Geometry check sheet. Reference: the model listing, model coordinates, mm. A direction names the side the tool comes from. Coordinates: 2 decimals unless noted, no trailing zeros. Write each loop counter-clockwise with the first axis right and the second up, starting at its lowest first coordinate (ties: lowest second). Pieces come first, ordered by that corner, then holes.
from build123d import *

# Parameters (mm, degrees)
SKETCH_1_W                      = 6
SKETCH_1_H                      = 20
EXTRUDE_1_DEPTH                 = 165
HOLE_WIZARD_G1_16_1_D           = 6.6
HOLE_WIZARD_G1_16_1_DEPTH       = 50
HOLE_WIZARD_G1_16_1_CSINK_D     = 7.773
HOLE_WIZARD_G1_16_1_CSINK_ANGLE = 90
HOLE_WIZARD_G1_16_1_TIP         = 1.982840043
SKETCH_5_W                      = 15
SKETCH_5_H                      = 20
EXTRUDE_2_DEPTH                 = 10
EXTRUDE_2_DEPTH_BACK            = 15
SKETCH_6_W                      = 5.5
SKETCH_6_H                      = 15
SKETCH_6_W_2                    = 4.5
CUT_EXTRUDE_1_DEPTH             = 32
SKETCH_7_W                      = 15
SKETCH_7_H                      = 18
CUT_EXTRUDE_2_DEPTH             = 14
SKETCH_8_R                      = 2
CUT_EXTRUDE_3_DEPTH             = 39
CUT_EXTRUDE_4_DEPTH             = 70


with BuildPart() as part:
    # 草图1 → 凸台-拉伸1 (new body)
    with BuildSketch(Plane.XY):
        Rectangle(SKETCH_1_W, SKETCH_1_H)
    extrude(amount=EXTRUDE_1_DEPTH)

    # G1/16 螺纹孔1
    with Locations(Plane(origin=(3, 0, 0), x_dir=(0, 0, -1), z_dir=(1, 0, 0))):
        with Locations((-5, 0)):
            CounterSinkHole(HOLE_WIZARD_G1_16_1_D / 2, HOLE_WIZARD_G1_16_1_CSINK_D / 2, depth=HOLE_WIZARD_G1_16_1_DEPTH, counter_sink_angle=HOLE_WIZARD_G1_16_1_CSINK_ANGLE)
            with Locations((0, 0, -(HOLE_WIZARD_G1_16_1_DEPTH + HOLE_WIZARD_G1_16_1_TIP / 2))):  # 118° drill point
                Cone(0, HOLE_WIZARD_G1_16_1_D / 2, HOLE_WIZARD_G1_16_1_TIP, mode=Mode.SUBTRACT)

    # 草图5 → 凸台-拉伸2 (add, two sides)
    with BuildSketch(Plane(origin=(3, 0, 0), x_dir=(0, 0, -1), z_dir=(1, 0, 0))) as extrude_2_sk:
        with Locations((-160.5, 0)):
            Rectangle(SKETCH_5_W, SKETCH_5_H)
    extrude(amount=EXTRUDE_2_DEPTH)
    extrude(extrude_2_sk.sketch, amount=-EXTRUDE_2_DEPTH_BACK)

    # 草图6 → 切除-拉伸1 (cut)
    with BuildSketch(Plane.XZ.offset(10)):
        with Locations((10.25, 160.5)):
            Rectangle(SKETCH_6_W, SKETCH_6_H)
        with Locations((-9.75, 160.5)):
            Rectangle(SKETCH_6_W_2, SKETCH_6_H)
    extrude(amount=-CUT_EXTRUDE_1_DEPTH, mode=Mode.SUBTRACT)

    # 草图7 → 切除-拉伸2 (cut)
    with BuildSketch(Plane.XY.offset(168)):
        Rectangle(SKETCH_7_W, SKETCH_7_H)
    extrude(amount=-CUT_EXTRUDE_2_DEPTH, mode=Mode.SUBTRACT)

    # 草图8 → 切除-拉伸3 (cut)
    with BuildSketch(Plane(origin=(0, 10, 0), x_dir=(1, 0, 0), z_dir=(0, 1, 0))):
        with Locations((0, -165)):
            Circle(SKETCH_8_R)
    extrude(amount=-CUT_EXTRUDE_3_DEPTH, mode=Mode.SUBTRACT)

    # 草图9 → 切除-拉伸4 (cut)
    with BuildSketch(Plane.ZY.offset(3)):
        Polygon((14.328441006, 1.918732887), (24.619003084, 1.918732887), (22.600253038, 5.415310533), (16.347191051, 5.415310533), align=None)
        Polygon((22.600253038, -5.415310533), (24.57465807, -1.995540703), (14.372786019, -1.995540703), (16.347191051, -5.415310533), align=None)
        Polygon((32.73389091, 1.918732887), (45.062363825, 1.918732887), (45.062363825, 3.558923578), (38.898127367, 7.117847156), (32.73389091, 3.558923578), align=None)
        Polygon((45.062363825, -3.558923578), (45.062363825, -1.995540703), (32.73389091, -1.995540703), (32.73389091, -3.558923578), (38.898127367, -7.117847156), align=None)
        Polygon((52.911163907, 1.918732887), (65.330427938, 1.918732887), (62.779502404, 6.337065517), (55.46208944, 6.337065517), align=None)
        Polygon((62.779502404, -6.337065517), (65.286082924, -1.995540703), (52.95550892, -1.995540703), (55.46208944, -6.337065517), align=None)
        Polygon((87.237271272, -3.558923578), (87.237271272, -1.995540703), (74.908798357, -1.995540703), (74.908798357, -3.558923578), (81.073034814, -7.117847156), align=None)
        Polygon((74.908798357, 1.918732887), (87.237271272, 1.918732887), (87.237271272, 3.558923578), (81.073034814, 7.117847156), (74.908798357, 3.558923578), align=None)
        Polygon((97.746948796, 1.918732887), (110.964476059, 1.918732887), (108.213984717, 6.682723636), (100.497440137, 6.682723636), align=None)
        Polygon((108.213984717, -6.682723636), (110.920131045, -1.995540703), (97.791293809, -1.995540703), (100.497440137, -6.682723636), align=None)
        Polygon((118.547188397, 1.918732887), (130.875661312, 1.918732887), (130.875661312, 3.558923578), (124.711424854, 7.117847156), (118.547188397, 3.558923578), align=None)
        Polygon((130.875661312, -3.558923578), (130.875661312, -1.995540703), (118.547188397, -1.995540703), (118.547188397, -3.558923578), (124.711424854, -7.117847156), align=None)
        Polygon((138.857505266, 1.918732887), (149.946330576, 1.918732887), (147.728014723, 5.760968652), (141.075821119, 5.760968652), align=None)
        Polygon((147.728014723, -5.760968652), (149.901985563, -1.995540703), (138.901850279, -1.995540703), (141.075821119, -5.760968652), align=None)
    extrude(amount=-CUT_EXTRUDE_4_DEPTH, mode=Mode.SUBTRACT)


solid = part.part
1. Access from +Z, -Z, +X, -X, +Y, -Y to the whole of each face (thin tool, end or side, straight path). Record for faces 1 (the flat face through (3, 0, 75)), 2 (the flat face through (0, 5.761, 144)), 3 (the flat face through (0, -9, 161)).
Computed values:
face 1: -Z, +X, +Y, -Y
face 2: +X, -X
face 3: +Z, +X, -X
2. Sectioned sample at D-D, the plane z = 165. Record the boundary of the cut face in (x, y), and give its area (3 significant figures).
Computed values:
outline: (-7.5, -10) - (-2, -10) - (-2, -9) - (-7.5, -9) - close; (-7.5, 9) - (-2, 9) - (-2, 10) - (-7.5, 10) - close; (2, -10) - (7.5, -10) - (7.5, -9) - (2, -9) - close; (2, 9) - (7.5, 9) - (7.5, 10) - (2, 10) - close
area: 22.0 mm2
3. Sectioned sample at A-A, the plane z = 5. Record the boundary of the cut face in (x, y), and give its area (3 significant figures).
Computed values:
outline: (-3, -10) - (3, -10) - (3, -3.89) - (2.41, -3.3) - (-3, -3.3) - close; (-3, 3.3) - (2.41, 3.3) - (3, 3.89) - (3, 10) - (-3, 10) - close
area: 80.1 mm2
4. Thickness scan on line 1 along Y through (x, z) = (0.5, 146.5); line 2 along Y through (x, z) = (-1.25, 61); line 3 along Z through (x, y) = (0, 9.7). Record the ranges inside material, lowest first.
Computed values:
line 1: y = -10 to -5.76, -2 to 1.92, 5.76 to 10
line 2: y = -10 to -6.34, -2 to 1.92, 6.34 to 10
line 3: z = 0 to 163, 167 to 168
5. Sectioned sample at B-B, the plane x = 4.5. Record the boundary of the cut face in (y, z), and give its area (3 significant figures).
Computed values:
outline: (-10, 153) - (10, 153) - (10, 168) - (9, 168) - (9, 154) - (-9, 154) - (-9, 168) - (-10, 168) - close
area: 48.0 mm2
6. Draft check along Z on faces 4 (the flat face through (-5, 0, 153)), 5 (the flat face through (0, 6.337, 59)), 6 (the flat face through (0, -10, 104)). Enter one of: released by +Z, released by -Z, zero draft, split by the parting line, or undercut.
Computed values:
face 4: released by -Z
face 5: undercut
face 6: zero draft
7. Gauge pin test, flat ends, axial feed: pin 1 Ø0.8 at (x, y) = (1, -2.5) entering from +Z; pin 2 Ø1.5 at (y, z) = (-6, 49) entering from +X; pin 3 Ø2 at (y, z) = (-2.5, 115) entering from -X. Record the tip position at first contact, or that the pin passes through.
Computed values:
pin 1: stops at z = 154
pin 2: stops at x = 3
pin 3: stops at x = -3
8. Sectioned sample at C-C, the plane z = 105.5. Record the boundary of the cut face in (x, y).
Computed values:
outline: (-3, -10) - (3, -10) - (3, -6.68) - (-3, -6.68) - close; (-3, -2) - (3, -2) - (3, 1.92) - (-3, 1.92) - close; (-3, 6.68) - (3, 6.68) - (3, 10) - (-3, 10) - close
